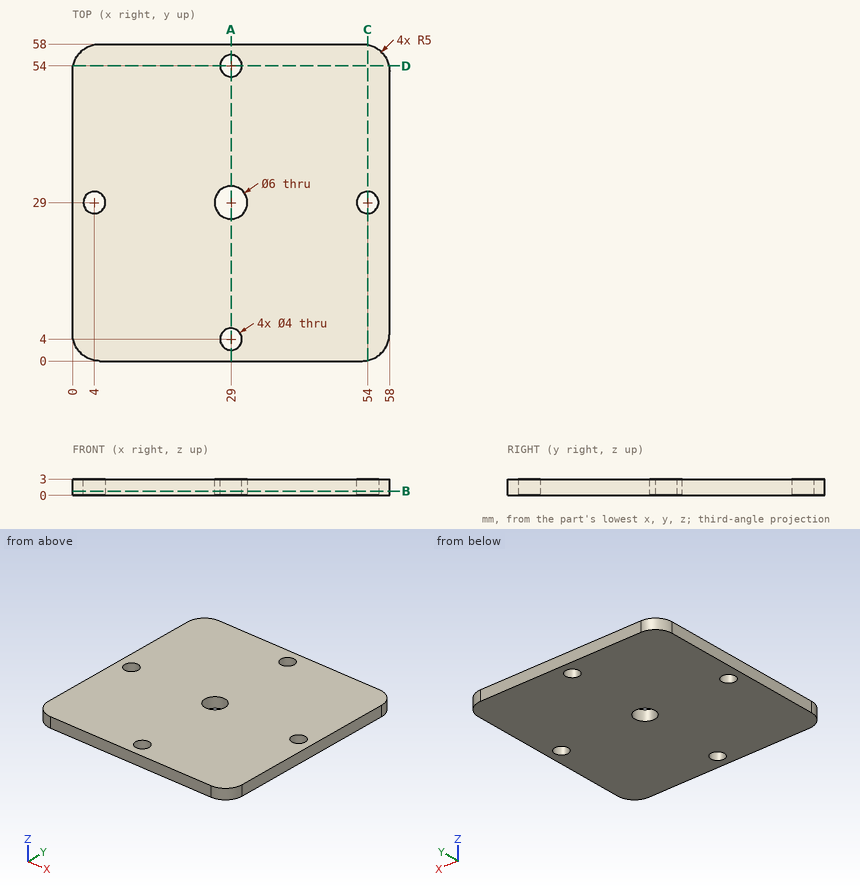
Geometry check sheet. Reference: drawing and pictorial views, mm from the part's lowest x, y, z. Coordinates: 2 decimals unless noted, no trailing zeros. Order: outer loops, then holes, each group sorted by start corner. A loop starts at its lowest first (then second) coordinate and runs counter-clockwise, first axis right, second up. Notation, with made-up numbers: M 58,-9.75 L 83,-9.75 A31 cw 83,24.25 Z; hole C 51,62 d11. An arc over 180 degrees is marked long. Write each question's results on one line, items separated by ' | '. Start each with the question number.
1. Material ranges on probe 1 along Y at (x, z) = (29, 2); probe 2 along X at (y, z) = (4, 1.2), recorded low to high.
2. Cross-section at C-C on x = 54. Record the cut outline in (y, z).
3. Cross-section at B-B on z = 0.8. Record the cut outline in (x, y).
4. Cross-section at A-A on x = 29. Record the cut outline in (y, z), and give its area (3 significant figures).
Checks:
1) probe 1: y = 0 to 2, 6 to 26, 32 to 52, 56 to 58 | probe 2: x = 0.1 to 27, 31 to 57.9
2) outline: M 0.1,0 L 27,0 L 27,3 L 0.1,3 Z; M 31,0 L 57.9,0 L 57.9,3 L 31,3 Z
3) outline: M 0,5 A5 ccw 5,0 L 53,0 A5 ccw 58,5 L 58,53 A5 ccw 53,58 L 5,58 A5 ccw 0,53 Z; hole C 4,29 d4; hole C 29,29 d6; hole C 29,4 d4; hole C 29,54 d4; hole C 54,29 d4
4) outline: M 0,0 L 2,0 L 2,3 L 0,3 Z; M 6,0 L 26,0 L 26,3 L 6,3 Z; M 32,0 L 52,0 L 52,3 L 32,3 Z; M 56,0 L 58,0 L 58,3 L 56,3 Z | area: 132 mm²
